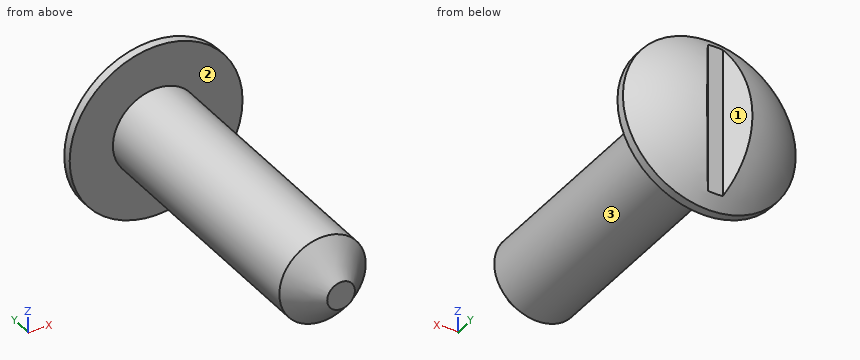
from build123d import *

# Parameters (mm, degrees)
DOME1_FACE_RADIUS       = 500
DOME1_HEIGHT            = 200
CUT_EXTRUDE1_DEPTH      = 2075.246851269
CUT_EXTRUDE1_DEPTH_BACK = 2075.246851269
CHAMFER5_SIZE           = 170


with BuildPart() as part:
    # Sketch1 → Revolve1 (revolve)
    with BuildSketch(Plane.XY, mode=Mode.PRIVATE) as revolve1_sk:
        Polygon((0, 0), (-250, 0), (-250, 1700), (-500, 1700), (-500, 1750), (0, 1750), align=None)
    revolve(revolve1_sk.sketch.rotate(Axis((0, 0, 0), (0, -1, 0)), 270), axis=Axis((0, 0, 0), (0, -1, 0)))

    # Dome1: a dome of height H over a round flat face of radius A is a cap of a sphere of radius (A * A + H * H) / (2 * H)
    dome1_r = (DOME1_FACE_RADIUS * DOME1_FACE_RADIUS + DOME1_HEIGHT * DOME1_HEIGHT) / (2 * DOME1_HEIGHT)
    dome1_base = Plane((0, 1750, 0), z_dir=(0, 1, 0))
    with Locations(dome1_base.offset(DOME1_HEIGHT - dome1_r)):
        dome1_ball = Sphere(dome1_r, mode=Mode.PRIVATE)
    add(split(dome1_ball, bisect_by=dome1_base, keep=Keep.TOP, mode=Mode.PRIVATE))

    # Sketch2 → Cut-Extrude1 (cut, two sides: drawn at the far end of the back side and taken through both)
    with BuildSketch(Plane.XY.offset(-CUT_EXTRUDE1_DEPTH_BACK)):
        Polygon((-2374.803234017, 5352.955339177), (-130.529221516, 1938.152944557), (-43.296369992, 1805.422739327), (43.296369992, 1805.422739327), (130.529221516, 1938.152944557), (2374.803234017, 5352.955339177), (2374.803234017, 13525.50481593), (-2374.803234017, 13525.50481593), align=None)
    extrude(amount=CUT_EXTRUDE1_DEPTH + CUT_EXTRUDE1_DEPTH_BACK, mode=Mode.SUBTRACT)

    # Chamfer5
    chamfer5_edges = [part.edges().sort_by_distance(p)[0] for p in [
        (0, 0, -250),
    ]]
    chamfer(chamfer5_edges, length=CHAMFER5_SIZE)


solid = part.part
Can you work these out from the model? Positions are in its coordinate system, mm. Face numbers are marked on the shaded views. Coordinates: 2 decimals unless noted, no trailing zeros. Order: outer loops, then holes, each group sorted by start corner. A loop starts at its lowest first (then second) coordinate and runs counter-clockwise, first axis right, second up. Notation, with made-up numbers: (52.5, 52.5) - (92.5, 52.5) arc R13 cw to (92.5, 76.5) - close; hole circle Ø10 at (-29.5, 5). An arc over 180 degrees is marked (long way). Answer as a JSON object with one key per item and string values. Group by question number.
Q1. Imagine slicing it at D-D (x = -430). Please give me the cut outline in (y, z).
Q2. I need wall thicknesses on line 1 (Z direction, x = 6, y = 1321.5); line 2 (Y direction, x = -106, z = 267); line 3 (Y direction, x = -269.5, z = 251). Which ranges of each line are inside material? Lowest first, please. Write a range as from..to.
Q3. Imagine slicing it at B-B (x = 0). Please give me the cut outline in (y, z), and give its area (3 significant figures).
Q4. We'd pull the mould along X, two halves only. Please class the marked faces 1, 2 and 3: +X half, -X half, draft (parallel to the pull), parting line (faces both ways), or undercut.
Q5. Will these pins go through, and if not, where does the flat tip stop? P1, Ø6, axis at x = 39.5, y = 866.5, coming from the -Z side; P2, Ø12, axis at x = -170, z = 21.5, coming from the -Y side; P3, Ø5, axis at x = 221, z = 245, coming from the +Y side.
Q6. Imagine slicing it at A-A (z = 0). Please give me the cut outline in (x, y).
Q7. Imagine slicing it at C-C (y = 540). Please give me the cut outline in (x, z).
Determined:
{
 "1": {"outline": "(1700, -255.15) - (1750, -255.15) arc R583.72 ccw to (1750, 255.15) - (1700, 255.15) - close"},
 "2": {"line 1": "z = -249.93..249.93", "line 2": "y = 1700..1890.66", "line 3": "y = 1700..1849.49"},
 "3": {"outline": "(0, -80) - (170, -250) - (1700, -250) - (1700, -500) - (1750, -500) arc R725 ccw to (1805.42, -434.44) - (1805.42, 434.44) arc R725 ccw to (1750, 500) - (1700, 500) - (1700, 250) - (170, 250) - (0, 80) - close", "area": "923,000 mm2"},
 "4": {"face 1": "undercut", "face 2": "draft", "face 3": "parting line"},
 "5": {"P1": "stops at z = -247.32", "P2": "stops at y = 85.35", "P3": "stops at y = 1871.84"},
 "6": {"outline": "(-500, 1700) - (-250, 1700) - (-250, 170) - (-80, 0) - (80, 0) - (250, 170) - (250, 1700) - (500, 1700) - (500, 1750) arc R725 ccw to (130.53, 1938.15) - (43.3, 1805.42) - (-43.3, 1805.42) - (-130.53, 1938.15) arc R725 ccw to (-500, 1750) - close"},
 "7": {"outline": "circle Ø500 at (0, 0)"}
}
